from build123d import *

# Parameters (mm, degrees)
SKETCH_1_W          = 6
SKETCH_1_H          = 40
SKETCH_1_R          = 1.6
EXTRUDE_1_DEPTH     = 2
CUT_EXTRUDE_1_DEPTH = 2
EXTRUDE_2_DEPTH     = 2


with BuildPart() as part:
    # 草图1 → 凸台-拉伸1 (new body)
    # profile 1 of 3: a face of its own
    with BuildSketch(Plane.XY):
        with Locations((-60.5, -1.75)):
            Rectangle(SKETCH_1_W, SKETCH_1_H)
        with Locations((-60.5, -6.75)):
            Circle(SKETCH_1_R, mode=Mode.SUBTRACT)
        with Locations((-60.5, 13.25)):
            Circle(SKETCH_1_R, mode=Mode.SUBTRACT)
    # profile 2 of 3: a face of its own
    with BuildSketch(Plane.XY):
        Polygon((-57.5, 18.25), (-57.5, -21.75), (57.5, -21.75), (57.5, 18.25), (63.5, 18.25), (63.5, 21.75), (-63.5, 21.75), (-63.5, 18.25), align=None)
        with Locations((-48.5, 18.75)):
            Circle(SKETCH_1_R, mode=Mode.SUBTRACT)
        with Locations((-23.5, 18.75)):
            Circle(SKETCH_1_R, mode=Mode.SUBTRACT)
        with Locations((23.5, 18.75)):
            Circle(SKETCH_1_R, mode=Mode.SUBTRACT)
        with Locations((48.5, 18.75)):
            Circle(SKETCH_1_R, mode=Mode.SUBTRACT)
    # profile 3 of 3: a face of its own
    with BuildSketch(Plane.XY):
        with Locations((60.5, -1.75)):
            Rectangle(SKETCH_1_W, SKETCH_1_H)
        with Locations((60.5, -6.75)):
            Circle(SKETCH_1_R, mode=Mode.SUBTRACT)
        with Locations((60.5, 13.25)):
            Circle(SKETCH_1_R, mode=Mode.SUBTRACT)
    extrude(amount=EXTRUDE_1_DEPTH)

    # 草图2 → 切除-拉伸1 (cut)
    with BuildSketch(Plane.XY.offset(2)):
        with BuildLine():
            Line((3.5, 12.75), (3.5, -13.75))
            ThreePointArc((3.5, -13.75), (0, -17.25), (-3.5, -13.75))
            Line((-3.5, -13.75), (-3.5, 12.75))
            ThreePointArc((-3.5, 12.75), (0, 16.25), (3.5, 12.75))
        make_face()
        with BuildLine():
            Line((14, 12.75), (14, -13.75))
            ThreePointArc((14, -13.75), (10.5, -17.25), (7, -13.75))
            Line((7, -13.75), (7, 12.75))
            ThreePointArc((7, 12.75), (10.5, 16.25), (14, 12.75))
        make_face()
        with BuildLine():
            Line((24.5, 12.75), (24.5, -13.75))
            ThreePointArc((24.5, -13.75), (21, -17.25), (17.5, -13.75))
            Line((17.5, -13.75), (17.5, 12.75))
            ThreePointArc((17.5, 12.75), (21, 16.25), (24.5, 12.75))
        make_face()
        with BuildLine():
            Line((35, 12.75), (35, -13.75))
            ThreePointArc((35, -13.75), (31.5, -17.25), (28, -13.75))
            Line((28, -13.75), (28, 12.75))
            ThreePointArc((28, 12.75), (31.5, 16.25), (35, 12.75))
        make_face()
        with BuildLine():
            Line((45.5, 12.75), (45.5, -13.75))
            ThreePointArc((45.5, -13.75), (42, -17.25), (38.5, -13.75))
            Line((38.5, -13.75), (38.5, 12.75))
            ThreePointArc((38.5, 12.75), (42, 16.25), (45.5, 12.75))
        make_face()
        with BuildLine():
            Line((-7, 12.75), (-7, -13.75))
            ThreePointArc((-7, -13.75), (-10.5, -17.25), (-14, -13.75))
            Line((-14, -13.75), (-14, 12.75))
            ThreePointArc((-14, 12.75), (-10.5, 16.25), (-7, 12.75))
        make_face()
        with BuildLine():
            Line((-17.5, 12.75), (-17.5, -13.75))
            ThreePointArc((-17.5, -13.75), (-21, -17.25), (-24.5, -13.75))
            Line((-24.5, -13.75), (-24.5, 12.75))
            ThreePointArc((-24.5, 12.75), (-21, 16.25), (-17.5, 12.75))
        make_face()
        with BuildLine():
            Line((-28, 12.75), (-28, -13.75))
            ThreePointArc((-28, -13.75), (-31.5, -17.25), (-35, -13.75))
            Line((-35, -13.75), (-35, 12.75))
            ThreePointArc((-35, 12.75), (-31.5, 16.25), (-28, 12.75))
        make_face()
        with BuildLine():
            Line((-38.5, 12.75), (-38.5, -13.75))
            ThreePointArc((-38.5, -13.75), (-42, -17.25), (-45.5, -13.75))
            Line((-45.5, -13.75), (-45.5, 12.75))
            ThreePointArc((-45.5, 12.75), (-42, 16.25), (-38.5, 12.75))
        make_face()
        with BuildLine():
            Line((-49, 12.75), (-49, -13.75))
            ThreePointArc((-49, -13.75), (-52.5, -17.25), (-56, -13.75))
            Line((-56, -13.75), (-56, 12.75))
            ThreePointArc((-56, 12.75), (-52.5, 16.25), (-49, 12.75))
        make_face()
        with BuildLine():
            Line((56, 12.75), (56, -13.75))
            ThreePointArc((56, -13.75), (52.5, -17.25), (49, -13.75))
            Line((49, -13.75), (49, 12.75))
            ThreePointArc((49, 12.75), (52.5, 16.25), (56, 12.75))
        make_face()
    extrude(amount=-CUT_EXTRUDE_1_DEPTH, mode=Mode.SUBTRACT)

    # 草图3 → 凸台-拉伸2 (add)
    with BuildSketch(Plane.XY.offset(2)):
        Polygon((49.5, -21.75), (49.5, -32.75), (61.5, -32.75), (56.5, -29.75), (56.5, -27.75), (61.5, -21.75), align=None)
    extrude(amount=-EXTRUDE_2_DEPTH)


solid = part.part
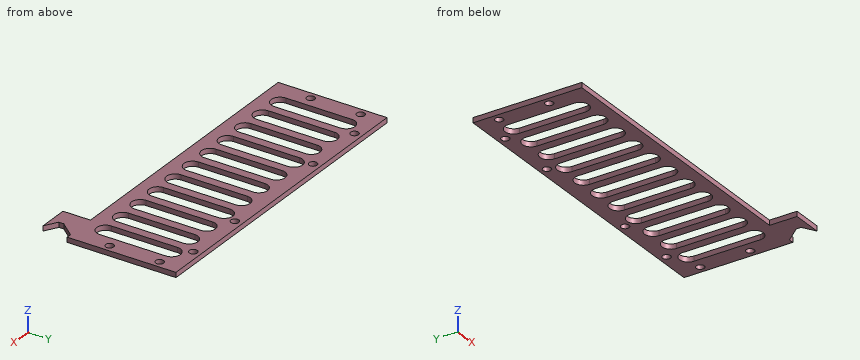
CAD build for the part. Positions are in the model's coordinates, mm. Coordinates: 2 decimals unless noted, no trailing zeros. Loops run counter-clockwise (first coordinate to the right, second up) from the corner with the lowest first, then second, coordinate; pieces in that order, holes last. Notation, with made-up numbers: (53, -27) - (97, -27) arc R19 ccw to (97, -4) - close; hole circle Ø2 at (-26, 0.25). An arc over 180 degrees is marked (long way). Write item = value, one per line. Start each with the question number.
Q1. Cut at A-A, the plane y = 18.75. List the corners of the cut face in (x, z).
Q2. Cut at B-B, the plane x = 0. List the corners of the cut face in (y, z), then the cut area to 3 significant figures.
Q3. Drill centre lines: L1, parallel to Y at x = -60.5, z = 1.15; L2, parallel to Y at x = 21, z = 0.4; L3, parallel to Y at x = 60.5, z = 1.3. Where is each one in solid material? Low to high.
Q4. Cut at D-D, the plane x = 52.5. List the corners of the cut face in (y, z), then the cut area to 3 significant figures.
Q5. Cut at C-C, the plane y = 8. Give the number of separate pieces and of enclosed holes in the cut face, then the cut area to 3 significant figures.
Computed:
q1.outline = (-63.5, 0) - (-50.1, 0) - (-50.1, 2) - (-63.5, 2) - close; (-46.9, 0) - (-25.1, 0) - (-25.1, 2) - (-46.9, 2) - close; (-21.9, 0) - (21.9, 0) - (21.9, 2) - (-21.9, 2) - close; (25.1, 0) - (46.9, 0) - (46.9, 2) - (25.1, 2) - close; (50.1, 0) - (63.5, 0) - (63.5, 2) - (50.1, 2) - close
q2.outline = (-21.75, 0) - (-17.25, 0) - (-17.25, 2) - (-21.75, 2) - close; (16.25, 0) - (21.75, 0) - (21.75, 2) - (16.25, 2) - close
q2.area = 20.0 mm²
q3.L1 = -21.75 to -8.35, -5.15 to 11.65, 14.85 to 21.75
q3.L2 = -21.75 to -17.25, 16.25 to 21.75
q3.L3 = -32.75 to -32.15, -22.95 to -8.35, -5.15 to 11.65, 14.85 to 21.75
q4.outline = (-32.75, 0) - (-17.25, 0) - (-17.25, 2) - (-32.75, 2) - close; (16.25, 0) - (21.75, 0) - (21.75, 2) - (16.25, 2) - close
q4.area = 42.0 mm²
q5.separate_pieces = 12
q5.enclosed_holes = 0
q5.area = 100 mm²
